Verification items for the finished model (mm, model axes). A direction names the side the tool comes from. Round coordinates to 2 decimals unless told otherwise and drop trailing zeros. Loops run counter-clockwise (first coordinate to the right, second up) from the corner with the lowest first, then second, coordinate; pieces in that order, holes last. Notation, with made-up numbers: M -26,-31 L -7,-31 A25 cw -7,-7 Z; hole C -29,57 d5. An arc over 180 degrees is marked long. Answer as CSV lines item,"result".
```python
from build123d import *

# Parameters (mm, degrees)
SKETCH1_W                 = 50
SKETCH1_H                 = 50
BOSS_EXTRUDE1_DEPTH       = 50
FILLET1_R                 = 1
F_3_0MM_DOWEL_HOLE1_D     = 3
F_3_0MM_DOWEL_HOLE1_DEPTH = 10
F_3_0MM_DOWEL_HOLE1_TIP   = 0.901290929
SKETCH5_R                 = 5
BOSS_EXTRUDE2_DEPTH       = 20


with BuildPart() as part:
    # Sketch1 → Boss-Extrude1 (new body)
    with BuildSketch(Plane(origin=(0, 0, 0), x_dir=(1, 0, 0), z_dir=(0, 1, 0))):
        Rectangle(SKETCH1_W, SKETCH1_H)
    extrude(amount=BOSS_EXTRUDE1_DEPTH)

    # Fillet1
    fillet1_edges = [part.edges().sort_by_distance(p)[0] for p in [
        (-25, 50, 0),
        (0, 50, 25),
        (25, 50, 0),
        (0, 0, 25),
        (-25, 0, 0),
        (0, 0, -25),
        (25, 0, 0),
        (0, 50, -25),
        (25, 25, 25),
        (-25, 25, 25),
        (-25, 25, -25),
        (25, 25, -25),
    ]]
    fillet(fillet1_edges, radius=FILLET1_R)

    # Ø3.0mm Dowel Hole1
    with Locations(Plane(origin=(0, 50, 0), x_dir=(1, 0, 0), z_dir=(0, 1, 0))):
        with Locations((-22.5, 22.5), (22.5, 22.5), (22.5, -22.5), (-22.5, -22.5)):
            Hole(F_3_0MM_DOWEL_HOLE1_D / 2, depth=F_3_0MM_DOWEL_HOLE1_DEPTH)
            with Locations((0, 0, -(F_3_0MM_DOWEL_HOLE1_DEPTH + F_3_0MM_DOWEL_HOLE1_TIP / 2))):  # 118° drill point
                Cone(0, F_3_0MM_DOWEL_HOLE1_D / 2, F_3_0MM_DOWEL_HOLE1_TIP, mode=Mode.SUBTRACT)

    # Sketch5 → Boss-Extrude2 (add)
    with BuildSketch(Plane(origin=(0, 50, 0), x_dir=(1, 0, 0), z_dir=(0, 1, 0))):
        with Locations(Location((0, 0, 0), (0, 0, 270))):
            Circle(SKETCH5_R)
    extrude(amount=BOSS_EXTRUDE2_DEPTH)


solid = part.part
```
1) Section check D-D (z = 14.5). Record the cut outline in (x, y).
Here are the results:
outline,"M -25,1 A1 ccw -24,0 L 24,0 A1 ccw 25,1 L 25,49 A1 ccw 24,50 L -24,50 A1 ccw -25,49 Z"
2) Section check C-C (x = 0). Record the cut outline in (y, z).
Here are the results:
outline,"M 0,-24 A1 ccw 1,-25 L 49,-25 A1 ccw 50,-24 L 50,-5 L 70,-5 L 70,5 L 50,5 L 50,24 A1 ccw 49,25 L 1,25 A1 ccw 0,24 Z"
3) Set-up check for faces 1 (the cylindrical face through (-21.39, 44.93, 21.49)), 2 (the flat face through (-23.7, 50, 23.64)): record each of +Z, -Z, +X, -X, +Y, -Y from which the full face is reachable in a straight line by a thin tool's end or side.
Here are the results:
face 1,"+Y"
face 2,"+Z, -Z, +X, -X, +Y"
4) Draft check along X on faces 3 (the cylindrical face through (-4.88, 59.86, -1.08)), 4 (the flat face through (-25, 25, 0)), 5 (the conical face through (22.748, 39.255, -22.578)). Enter one of: +X half, -X half, draft (parallel to the pull), parting line (faces both ways), or undercut.
Here are the results:
face 3,"parting line"
face 4,"-X half"
face 5,"undercut"
5) Material ranges on probe 1 along Z at (x, y) = (-22.5, 47); probe 2 along X at (y, z) = (43, -22), recorded low to high.
Here are the results:
probe 1,"z = -25 to -24, -21 to 21, 24 to 25"
probe 2,"x = -25 to -23.91, -21.09 to 21.09, 23.91 to 25"
6) Section check B-B (z = 0). Record the cut outline in (x, y).
Here are the results:
outline,"M -25,1 A1 ccw -24,0 L 24,0 A1 ccw 25,1 L 25,49 A1 ccw 24,50 L 5,50 L 5,70 L -5,70 L -5,50 L -24,50 A1 ccw -25,49 Z"
7) Go/stop test with flat-tipped pins: pin 1 (4 mm diameter, centred on x = 5, z = -3, fed in from +Y); pin 2 (1.5 mm diameter, centred on y = 55, z = 6.5, fed in from -X); pin 3 (1.6 mm diameter, centred on x = 23.5, z = 23.5, fed in from +Y); pin 4 (2.5 mm diameter, centred on x = -22.5, z = -22.5, fed in from +Y). Record where each tip stops, or that it passes through.
Here are the results:
pin 1,"stops at y = 70"
pin 2,"passes through"
pin 3,"stops at y = 50"
pin 4,"stops at y = 39.85"
8) Section check A-A (x = -20). Record the cut outline in (y, z), plus the area to 3 significant figures.
Here are the results:
outline,"M 0,-24 A1 ccw 1,-25 L 49,-25 A1 ccw 50,-24 L 50,24 A1 ccw 49,25 L 1,25 A1 ccw 0,24 Z"
area,"2,500 mm^2"
